Source: CAD feature listing. Evaluate the final solid. Frame: model axes, mm. A direction names the side the tool comes from. Give positions to 0.01 mm unless a question says otherwise; leave off trailing zeros. Loops run counter-clockwise (first coordinate to the right, second up) from the corner with the lowest first, then second, coordinate; pieces in that order, holes last. Notation, with made-up numbers: (41, -13) -> (94, -13) arc R22 cw to (94, 22) -> close; hole circle Ø10 at (18, 65.5). An arc over 180 degrees is marked (long way). Return JSON: item names as keys, results as strings. Group by question number.
```python
from build123d import *

# Parameters (mm, degrees)
BOSS_EXTRUDE1_DEPTH = 6.35
SKETCH2_R           = 3.5
CUT_EXTRUDE1_DEPTH  = 7.35
SKETCH3_W           = 14.231578179
SKETCH3_H           = 34.511577086
CUT_EXTRUDE2_DEPTH  = 25


with BuildPart() as part:
    # Sketch1 → Boss-Extrude1 (new body)
    with BuildSketch(Plane.XY):
        Polygon((12.7, 0), (-12.7, 0), (-12.7, 50.8), (-63.1, 50.8), (-63.1, 76.2), (12.7, 76.2), (12.7, 50.8), align=None)
    extrude(amount=BOSS_EXTRUDE1_DEPTH)

    # Sketch2 → Cut-Extrude1 (cut, through all)
    with BuildSketch(Plane.XY.offset(6.35)):
        with Locations((0, 63.5)):
            Circle(SKETCH2_R)
        with Locations((-25.4, 63.5)):
            Circle(SKETCH2_R)
        with Locations((0, 38.1)):
            Circle(SKETCH2_R)
        with Locations((0, 12.7)):
            Circle(SKETCH2_R)
        with Locations((-50.8, 63.5)):
            Circle(SKETCH2_R)
    extrude(amount=-CUT_EXTRUDE1_DEPTH, mode=Mode.SUBTRACT)

    # Sketch3 → Cut-Extrude2 (cut)
    with BuildSketch(Plane.ZY.offset(63.1)):
        with Locations((3.571370897, 64.988127963)):
            Rectangle(SKETCH3_W, SKETCH3_H)
    extrude(amount=-CUT_EXTRUDE2_DEPTH, mode=Mode.SUBTRACT)


solid = part.part
```
1) Cut plane C-C on z = 4. Return loops of the section in (x, y).
2) Cut plane B-B on x = -25.4. Return loops of the section in (y, z).
3) Material intervals for line 1 (Y direction, x = 0, z = 4.5); line 2 (X direction, y = 66, z = 2.5); line 3 (Y direction, x = -25.4, z = 2), sorted ascending.
4) Cut plane D-D on y = 12.7. Return loops of the section in (x, z), then the cut area to 3 significant figures.
5) Mould query, pull axis Y, two halves, no side actions, for faces 3 (the face through (-7, 47, 0)), 4 (the face through (-0.46, 16.17, 3.22)), 5 (the face through (-25, 50.8, 3)). Classes: released by +Y, released by -Y, zero draft, split by the parting line, or undercut.
6) Reachability of faces 1 (the face through (-12.7, 25, 3)), 2 (the face through (0, 0, 3)) from +Z, -Z, +X, -X, +Y, -Y: full face, straight path, thin tool, end or side. Return the list, or none.
7) Cut plane A-A on y = 63.5. Return loops of the section in (x, z).
8) Contact query for a flat-ended pin moving along its axis: P1, Ø1, axis at x = -6.5, y = 48, coming from the -Z side. Output: stop coordinate, or through.
Calculated:
{
 "1": {"outline": "(-38.1, 50.8) -> (-12.7, 50.8) -> (-12.7, 0) -> (12.7, 0) -> (12.7, 76.2) -> (-38.1, 76.2) -> close; hole circle Ø7 at (-25.4, 63.5); hole circle Ø7 at (0, 12.7); hole circle Ø7 at (0, 38.1); hole circle Ø7 at (0, 63.5)"},
 "2": {"outline": "(50.8, 0) -> (60, 0) -> (60, 6.35) -> (50.8, 6.35) -> close; (67, 0) -> (76.2, 0) -> (76.2, 6.35) -> (67, 6.35) -> close"},
 "3": {"line 1": "0 to 9.2, 16.2 to 34.6, 41.6 to 60, 67 to 76.2", "line 2": "-38.1 to -27.85, -22.95 to -2.45, 2.45 to 12.7", "line 3": "50.8 to 60, 67 to 76.2"},
 "4": {"outline": "(-12.7, 0) -> (-3.5, 0) -> (-3.5, 6.35) -> (-12.7, 6.35) -> close; (3.5, 0) -> (12.7, 0) -> (12.7, 6.35) -> (3.5, 6.35) -> close", "area": "117 mm2"},
 "5": {"face 3": "zero draft", "face 4": "undercut", "face 5": "released by -Y"},
 "6": {"face 1": "+Z, -Z, -X, -Y", "face 2": "+Z, -Z, +X, -X, -Y"},
 "7": {"outline": "(-38.1, 0) -> (-28.9, 0) -> (-28.9, 6.35) -> (-38.1, 6.35) -> close; (-21.9, 0) -> (-3.5, 0) -> (-3.5, 6.35) -> (-21.9, 6.35) -> close; (3.5, 0) -> (12.7, 0) -> (12.7, 6.35) -> (3.5, 6.35) -> close"},
 "8": {"P1": "z = 0"}
}
